Can you work these out from the model? Positions are in its coordinate system, mm. Face numbers are marked on the shaded views. A direction names the side the tool comes from. Coordinates: 2 decimals unless noted, no trailing zeros. Loops run counter-clockwise (first coordinate to the right, second up) from the corner with the lowest first, then second, coordinate; pieces in that order, holes last. Notation, with made-up numbers: M -25,88 L -6,88 A32 ccw -6,119 Z; hole C 67,37 d11. An arc over 180 degrees is marked long. Answer as a JSON object with one key per item and string values. Group by question number.
Item 1: I'm going to push flat-ended pins straight in: pin 1 Ø1 at (y, z) = (-1, -5) entering from -X; pin 2 Ø2 at (x, z) = (38, -4) entering from -Y; pin 3 Ø2.5 at (x, z) = (37, -3.5) entering from -Y; pin 4 Ø0.6 at (y, z) = (-1, -2.5) entering from +X. Where does each tip first touch, or does it pass through?
Item 2: Suppose I cut it at D-D (z = -1.25). Write out the boundary of the cut face in (x, y).
Item 3: Which directions (+Z, -Z, +X, -X, +Y, -Y) give clear straight access to the entire face, cutting with the end or side of a thin tool? Please do the marked faces 5, 6, 7, 8 and 9.
Item 4: Suppose I cut it at B-B (x = 5). Write out the boundary of the cut face in (y, z) (3 decimals).
Item 5: We'd pull the mould along Z, two halves only. Please class the marked faces 1, 2, 3 and 4: +Z half, -Z half, draft (parallel to the pull), parting line (faces both ways), or undercut.
Item 6: Suppose I cut it at A-A (z = -3.5). Write out the boundary of the cut face in (x, y) (3 decimals), then the cut area to 4 significant figures.
Item 7: Suppose I cut it at C-C (y = 2). Write out the boundary of the cut face in (x, z) (3 decimals), then the cut area to 3 significant figures.
Item 8: If I drill on line 1 (X direction, y = 1.8, z = -3.5) (3 decimals); line 2 (X direction, y = 6.75, z = -3.25); line 3 (X direction, y = 3, z = -4.5), over which ranges is the centre line in solid material (lowest first)?
```python
from build123d import *

# Parameters (mm, degrees)
SKETCH1_W            = 42
SKETCH1_H            = 7
RISER_DEPTH          = 7
SKETCH2_R            = 1.475
MOUNTING_HOLES_DEPTH = 44.150898021
SKETCH4_W            = 40
SKETCH4_H            = 6
RECESS_3_SIDES_DEPTH = 2
SKETCH5_W            = 22
SKETCH5_H            = 7
ALIGNMENT_TAB_DEPTH  = 2


with BuildPart() as part:
    # Sketch1 → Riser (new body)
    with BuildSketch(Plane(origin=(0, 0, 0), x_dir=(1, 0, 0), z_dir=(0, 1, 0))):
        with Locations((21, 3.5)):
            Rectangle(SKETCH1_W, SKETCH1_H)
    extrude(amount=RISER_DEPTH)

    # Sketch2 → Mounting Holes (cut, through all)
    with BuildSketch(Plane.XZ):
        with Locations(Location((5, -3.5, 0), (0, 0, 270))):
            Circle(SKETCH2_R)
        with Locations(Location((37, -3.5, 0), (0, 0, 90))):
            Circle(SKETCH2_R)
    extrude(amount=-MOUNTING_HOLES_DEPTH, mode=Mode.SUBTRACT)

    # Sketch4 → Recess (3-Sides) (cut)
    with BuildSketch(Plane(origin=(0, 7, 0), x_dir=(1, 0, 0), z_dir=(0, 1, 0))):
        with Locations((21, 3)):
            Rectangle(SKETCH4_W, SKETCH4_H)
    extrude(amount=-RECESS_3_SIDES_DEPTH, mode=Mode.SUBTRACT)

    # Sketch5 → Alignment Tab (add)
    with BuildSketch(Plane.XZ):
        with Locations((21, -3.5)):
            Rectangle(SKETCH5_W, SKETCH5_H)
    extrude(amount=ALIGNMENT_TAB_DEPTH)


solid = part.part
```
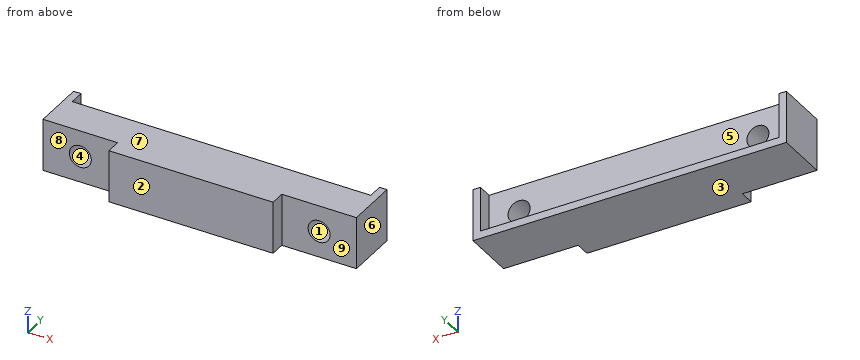
From the geometry:
{
 "1": {"pin 1": "x = 10", "pin 2": "y = 0", "pin 3": "through", "pin 4": "x = 32"},
 "2": {"outline": "M 0,0 L 10,0 L 10,-2 L 32,-2 L 32,0 L 42,0 L 42,7 L 41,7 L 41,5 L 1,5 L 1,7 L 0,7 Z"},
 "3": {"face 5": "+Z, +Y", "face 6": "+Z, -Z, +X, +Y, -Y", "face 7": "+Z, +X, -X, +Y, -Y", "face 8": "+Z, -Z, -X, -Y", "face 9": "+Z, -Z, +X, -Y"},
 "4": {"outline": "M 0,-7 L 7,-7 L 7,-6 L 5,-6 L 5,-4.975 L 0,-4.975 Z; M 0,-2.025 L 5,-2.025 L 5,0 L 0,0 Z"},
 "5": {"face 1": "undercut", "face 2": "draft", "face 3": "-Z half", "face 4": "undercut"},
 "6": {"outline": "M 0,0 L 3.525,0 L 3.525,5 L 1,5 L 1,7 L 0,7 Z; M 6.475,0 L 10,0 L 10,-2 L 32,-2 L 32,0 L 35.525,0 L 35.525,5 L 6.475,5 Z; M 38.475,0 L 42,0 L 42,7 L 41,7 L 41,5 L 38.475,5 Z", "area": "228.5 mm2"},
 "7": {"outline": "M 0,-7 L 42,-7 L 42,0 L 0,0 Z; hole C 5,-3.5 d2.95; hole C 37,-3.5 d2.95", "area": "280 mm2"},
 "8": {"line 1": "0 to 3.525, 6.475 to 35.525, 38.475 to 42", "line 2": "0 to 1, 41 to 42", "line 3": "0 to 3.92, 6.08 to 35.92, 38.08 to 42"}
}
